from build123d import *

# Parameters (mm, degrees)
ESBO_O1_W                = 40.5
ESBO_O1_H                = 35.5
RESSALTO_EXTRUS_O1_DEPTH = 20
RESSALTO_EXTRUS_O2_DEPTH = 2
ESBO_O3_W                = 18
ESBO_O3_H                = 2.499999999
RESSALTO_EXTRUS_O3_DEPTH = 7
CORTE_EXTRUS_O1_DEPTH    = 11.500000003
CORTE_EXTRUS_O2_DEPTH    = 11.500000003
RESSALTO_EXTRUS_O4_DEPTH = 2
ESBO_O7_W                = 18
ESBO_O7_H                = 2.499999994
RESSALTO_EXTRUS_O5_DEPTH = 7
CORTE_EXTRUS_O3_DEPTH    = 30.499999991
CORTE_EXTRUS_O4_DEPTH    = 30.499999991
ESBO_O10_W               = 2.25
ESBO_O10_H               = 2.5
ESBO_O11_W               = 2.25
ESBO_O11_H               = 2.5
ESBO_O12_W               = 2.25
ESBO_O12_H               = 2.5
ESBO_O13_W               = 2.25
ESBO_O13_H               = 2.5
ESBO_O15_R               = 2.96
ESBO_O15_R_2             = 1.15
RESSALTO_EXTRUS_O6_DEPTH = 4


with BuildPart() as part:
    # Esboço1 → Ressalto-extrusão1 (new body)
    with BuildSketch(Plane(origin=(0, 0, -10), x_dir=(-1, 0, 0), z_dir=(0, 0, -1))):
        with Locations((0, 17.75)):
            Rectangle(ESBO_O1_W, ESBO_O1_H)
    extrude(amount=-RESSALTO_EXTRUS_O1_DEPTH)

    # Esboço2 → Ressalto-extrusão2 (add)
    with BuildSketch(Plane(origin=(0, 35.5, 0), x_dir=(-1, 0, 0), z_dir=(0, 1, 0))):
        with BuildLine():
            Line((-14.25, 9), (5.75, 9))
            ThreePointArc((5.75, 9), (20.108898944, -1e-09), (5.75, -9))
            Line((5.75, -9), (-14.25, -9))
            Line((-14.25, -9), (-14.25, 9))
        make_face()
    extrude(amount=RESSALTO_EXTRUS_O2_DEPTH)

    # Esboço3 → Ressalto-extrusão3 (add)
    with BuildSketch(Plane(origin=(20.25, 0, 0), x_dir=(0, 0, -1), z_dir=(1, 0, 0))):
        with Locations((0, 28.249999997)):
            Rectangle(ESBO_O3_W, ESBO_O3_H)
    extrude(amount=RESSALTO_EXTRUS_O3_DEPTH)

    # Esboço4 → Corte-extrusão1 (cut, through all)
    with BuildSketch(Plane.XZ.offset(-26.999999997)):
        with BuildLine():
            Line((27.25, 3.25), (27.25, 6.25))
            Line((27.25, 6.25), (26.177050983, 6.25))
            ThreePointArc((26.177050983, 6.25), (26.75, 4.75), (26.177050983, 3.25))
            Line((26.177050983, 3.25), (27.25, 3.25))
        make_face()
    extrude(amount=-CORTE_EXTRUS_O1_DEPTH, mode=Mode.SUBTRACT)

    # Esboço5 → Corte-extrusão2 (cut, through all)
    with BuildSketch(Plane.XZ.offset(-26.999999997)):
        with BuildLine():
            Line((27.25, -6.25), (27.25, -3.25))
            Line((27.25, -3.25), (26.177050983, -3.25))
            ThreePointArc((26.177050983, -3.25), (26.75, -4.75), (26.177050983, -6.25))
            Line((26.177050983, -6.25), (27.25, -6.25))
        make_face()
    extrude(amount=-CORTE_EXTRUS_O2_DEPTH, mode=Mode.SUBTRACT)

    # Esboço6 → Ressalto-extrusão4 (add)
    with BuildSketch(Plane(origin=(0, 35.5, 0), x_dir=(-1, 0, 0), z_dir=(0, 1, 0))):
        with BuildLine():
            Line((-14.249999993, 4.8), (-14.249999993, -4.800000003))
            ThreePointArc((-14.249999993, -4.800000003), (-16.649999996, -1e-09), (-14.249999993, 4.8))
        make_face()
    extrude(amount=RESSALTO_EXTRUS_O4_DEPTH)

    # Esboço7 → Ressalto-extrusão5 (add)
    with BuildSketch(Plane.ZY.offset(20.25)):
        with Locations((0, 28.249999994)):
            Rectangle(ESBO_O7_W, ESBO_O7_H)
    extrude(amount=RESSALTO_EXTRUS_O5_DEPTH)

    # Esboço8 → Corte-extrusão3 (cut, through all)
    with BuildSketch(Plane(origin=(0, 29.499999991, 0), x_dir=(-1, 0, 0), z_dir=(0, 1, 0))):
        with BuildLine():
            Line((27.25, 6.25), (26.177050983, 6.25))
            ThreePointArc((26.177050983, 6.25), (26.75, 4.75), (26.177050983, 3.25))
            Line((26.177050983, 3.25), (27.25, 3.25))
            Line((27.25, 3.25), (27.25, 6.25))
        make_face()
    extrude(amount=-CORTE_EXTRUS_O3_DEPTH, mode=Mode.SUBTRACT)

    # Esboço9 → Corte-extrusão4 (cut, through all)
    with BuildSketch(Plane(origin=(0, 29.499999991, 0), x_dir=(-1, 0, 0), z_dir=(0, 1, 0))):
        with BuildLine():
            Line((27.25, -6.25), (27.25, -3.25))
            Line((27.25, -3.25), (26.177050983, -3.25))
            ThreePointArc((26.177050983, -3.25), (26.75, -4.75), (26.177050983, -6.25))
            Line((26.177050983, -6.25), (27.25, -6.25))
        make_face()
    extrude(amount=-CORTE_EXTRUS_O4_DEPTH, mode=Mode.SUBTRACT)

    # Esboço10 → Corte-Revolução1 (revolve, cut)
    with BuildSketch(Plane.XY.offset(4.75)):
        with Locations((-23.375, 28.25)):
            Rectangle(ESBO_O10_W, ESBO_O10_H)
    revolve(axis=Axis((-24.5, 29.5, 4.75), (0, -1, 0)), mode=Mode.SUBTRACT)

    # Esboço11 → Corte-Revolução2 (revolve, cut)
    with BuildSketch(Plane.XY.offset(-4.75)):
        with Locations((-23.375, 28.25)):
            Rectangle(ESBO_O11_W, ESBO_O11_H)
    revolve(axis=Axis((-24.5, 29.5, -4.75), (0, -1, 0)), mode=Mode.SUBTRACT)

    # Esboço12 → Corte-Revolução3 (revolve, cut)
    with BuildSketch(Plane.XY.offset(-4.75)):
        with Locations((25.625, 28.25)):
            Rectangle(ESBO_O12_W, ESBO_O12_H)
    revolve(axis=Axis((24.5, 29.5, -4.75), (0, -1, 0)), mode=Mode.SUBTRACT)

    # Esboço13 → Corte-Revolução4 (revolve, cut)
    with BuildSketch(Plane.XY.offset(4.75)):
        with Locations((25.625, 28.25)):
            Rectangle(ESBO_O13_W, ESBO_O13_H)
    revolve(axis=Axis((24.5, 29.5, 4.75), (0, -1, 0)), mode=Mode.SUBTRACT)

    # Esboço14 → Revolução1 (revolve)
    with BuildSketch(Plane.XY):
        Polygon((-4.533898944, 39), (-10.108898944, 39), (-10.108898944, 37.5), (-3.708898944, 37.5), (-3.708898944, 38.5), (-4.533898944, 38.5), align=None)
    revolve(axis=Axis((-10.108898944, 39, 0), (0, -1, 0)))

    # Esboço15 → Ressalto-extrusão6 (add)
    with BuildSketch(Plane(origin=(0, 39, 0), x_dir=(1, 0, 0), z_dir=(0, 1, 0))):
        with Locations((-10.108898944, 0)):
            Circle(ESBO_O15_R)
        with Locations((-10.108898944, 0)):
            Circle(ESBO_O15_R_2, mode=Mode.SUBTRACT)
    extrude(amount=RESSALTO_EXTRUS_O6_DEPTH)


solid = part.part
Input: part model. Units: mm. Frame: model coordinates. A direction names the side the tool comes from. Give positions to 0.01 mm unless a question says otherwise; leave off trailing zeros. Order: outer loops, then holes, each group sorted by start corner. A loop starts at its lowest first (then second) coordinate and runs counter-clockwise, first axis right, second up.
Q1. Contact query for flat-ended pins moving along their axis: pin 1 Ø1.6 at (y, z) = (36, 7) entering from +X; pin 2 Ø12 at (y, z) = (15.5, 0.5) entering from -X; pin 3 Ø0.5 at (x, y) = (27, 29) entering from -Z. Output: stop coordinate, or through.
Checked values:
pin 1: stops at x = 20.25
pin 2: stops at x = -20.25
pin 3: stops at z = -9
Q2. Set-up query: faces 4 (the flat face through (4, 36, -9)), 5 (the flat face through (24, 28, 9)), 6 (the flat face through (-23, 27, 0)), 7 (the flat face through (14.25, 36, 7)). Return all of +Z, -Z, +X, -X, +Y, -Y with unobstructed straight access to the full face (end or side cutting, diameter ignored); none if empty.
Checked values:
face 4: -Z, +X, +Y
face 5: +Z, +X, +Y, -Y
face 6: +Z, -Z, -X, -Y
face 7: +Z, +X, +Y
Q3. Section C-C on x = -2. Output: boundary loops of the cut face in (y, z), and give its area (3 significant figures).
Checked values:
outline: (0, -10) - (35.5, -10) - (35.5, -9) - (37.5, -9) - (37.5, 9) - (35.5, 9) - (35.5, 10) - (0, 10) - close
area: 746 mm2
Q4. Draft query along X for faces 1 (the cylindrical face through (-22.25, 28.27, 4.67)), 2 (the flat face through (-23, 29.5, 0)), 3 (the cylindrical face through (-4.004, 38.007, 1.922)). Return one class per face: +X half, -X half, draft (parallel to the pull), parting line (faces both ways), or undercut.
Checked values:
face 1: undercut
face 2: draft
face 3: parting line
Q5. Ray query, probe 1 along Z at (x, y) = (24.5, 28.55); probe 2 along Y at (x, z) = (22, 6); probe 3 along X at (y, z) = (40.9, 0). Return the intervals inside material, ascending.
Checked values:
probe 1: z = -9 to -7, -2.5 to 2.5, 7 to 9
probe 2: y = 27 to 29.5
probe 3: x = -13.07 to -11.26, -8.96 to -7.15
Q6. Section D-D on y = 10.5. Output: boundary loops of the cut face in (x, z).
Checked values:
outline: (-20.25, -10) - (20.25, -10) - (20.25, 10) - (-20.25, 10) - close
Q7. Section A-A on x = 24.5. Output: boundary loops of the cut face in (y, z).
Checked values:
outline: (27, -9) - (29.5, -9) - (29.5, -7) - (27, -7) - close; (27, -2.5) - (29.5, -2.5) - (29.5, 2.5) - (27, 2.5) - close; (27, 7) - (29.5, 7) - (29.5, 9) - (27, 9) - close
